Autodesk Inventor part; units mm, degrees
ref_plane "YZ Plane" through (0, 0, 0) normal (1, 0, 0) x (0, 1, 0)
ref_plane "XZ Plane" through (0, 0, 0) normal (0, 1, 0) x (-1, 0, 0)
ref_plane "XY Plane" through (0, 0, 0) normal (0, 0, 1) x (1, 0, 0)
sketch "Sketch1" plane through (0, 0, 0) normal (1, 0, 0) x (0, 1, 0)
  circle A0 centre (0, 0) radius 4.7625
  line L0 (0, 0) -> (-76.2, 0) construction
  circle A1 centre (0, 0) radius 19.05
  line L1 (-4.7625, 18.4451) -> (-76.2, 0)
  line L2 (-76.2, 0) -> (-76.2, -114.3)
  circle A2 centre (0, 0) radius 76.2 construction
  line L3 (-76.2, -114.3) -> (-41.275, -114.3)
  line L4 (-41.275, -114.3) -> (-41.275, -69.85)
  line L5 (-41.275, -69.85) -> (-76.2, -49.686)
  line L6 (-41.275, -69.85) -> (13.6667, -13.2712)
  line L7 (-52.6181, -63.301) -> (-7.9567, -17.3088)
  line L8 (-66.675, -9.525) -> (-66.675, -55.1853)
  line L9 (-46.0375, -78.0989) -> (-76.2, -60.6846)
  line L10 (-46.0375, -78.0989) -> (-46.0375, -106.3625)
  line L11 (-46.0375, -106.3625) -> (-69.85, -106.3625)
  line L12 (-69.85, -106.3625) -> (-69.85, -64.3507)
  line L13 (-66.675, -9.525) -> (-64.7847, -9.525)
  line L14 (-64.7847, -9.525) -> (-16.4978, -9.525)
  line L15 (-76.2, 0) -> (-41.275, 0)
  line L16 (-41.275, 0) -> (-41.275, 25.4) construction
  line L17 (-41.275, 25.4) -> (-76.2, 25.4) construction
  line L18 (-76.2, 25.4) -> (-76.2, 0)
  line L19 (-41.275, 0) -> (-76.2, 25.4)
  point P0 (-50.4255, 6.6549)
  dimension "d0" = 9.525
  dimension "d1" = 76.2
  dimension "d2" = 38.1
  dimension "d3" = 114.3
  dimension "d4" = 152.4
  dimension "d5" = 34.925
  dimension "d6" = 44.45
  dimension "d7" = 60
  dimension "d9" = 12.7
  dimension "d10" = 9.525
  dimension "d11" = 9.525
  dimension "d12" = 7.9375
  dimension "d13" = 6.35
  dimension "d14" = 4.7625
  dimension "d17" = 9.525
  dimension "d19" = 34.925
  dimension "d20" = 25.4
extrude "Extrusion1" add sketch "Sketch1" along normal blind 6.35 contours A1 | A1 L14 L13 L8 L5 L2 L15 L19 L1 | L6 L5 L7 A1 | L19 L15 L1 | L1 L18 L19 | L4 L3 L2 L5
fillet "Fillet1" radius 6.35 10 edges at (3.175, -7.9567, -17.3088) (3.175, -16.4978, -9.525) (3.175, -52.6181, -63.301) (3.175, -66.675, -9.525) (3.175, -66.675, -55.1853) (3.175, -69.85, -64.3507) (3.175, -46.0375, -78.0989) (3.175, -46.0375, -106.3625) (3.175, -69.85, -106.3625) (3.175, -41.275, -69.85)
fillet "Fillet2" radius 6.35 2 edges at (3.175, -76.2, 25.4) (3.175, -50.4255, 6.6549)
sketch "Sketch2" plane through (6.35, 0, 0) normal (1, 0, 0) x (0, 0, -1)
  circle A0 centre (0, 0) radius 4.7625
  circle A1 centre (0, 0) radius 11.1125
  dimension "d24" = 22.225
extrude "Extrusion2" cut sketch "Sketch2" against normal blind 1.5875 contours A0 | A1
equation "\"d9\" = d8"
properties part number "Upright" material "Aluminum 6061"
Work out the finished part from the listing and answer in its coordinate system (mm). A direction names the side the tool comes from. Round coordinates to 2 decimals unless told otherwise and drop trailing zeros. Order: outer loops, then holes, each group sorted by start corner. A loop starts at its lowest first (then second) coordinate and runs counter-clockwise, first axis right, second up. Notation, with made-up numbers: M 20,80 L 76,80 A25 cw 76,97 Z; hole C -27.5,-14.5 d9. An arc over 180 degrees is marked long. Put each result on its own line as item: value. Start each with the question number.
Q1. Section D-D, the plane z = 0 is taken. Write down the section's boundary in (x, y), and give its area (3 significant figures).
Q2. Straight lines are drawn through the part: L1, parallel to Z at x = 1.75, y = -64; L2, parallel to Y at x = 5.1, z = 0; L3, parallel to Z at x = 5.5, y = -57.5 (1 decimal). For each, find the intervals that lie inside material, in ascending order. Write a range as [from, to].
Q3. Section C-C, the plane x = 1 is taken. Give the number of separate pieces and of enclosed holes in the cut face, and give its area (3 significant figures).
Q4. Section B-B, the plane y = 0 is taken. Write down the section's boundary in (x, z).
Q5. Flat-ended cylindrical pins translate along their axes: pin 1 (3 mm diameter, centred on x = 5, y = -62, fed in from +Z); pin 2 (3 mm diameter, centred on x = 5.5, z = -97.5, fed in from +Y) (3 decimals); pin 3 (3 mm diameter, centred on x = 2, y = -57, fed in from +Z). Find the tip coordinate at first contact, or state that the pin passes through.
Q6. For a pull along Y with two mould halves and no side action, classify faces 1 (the cylindrical face through (3.219, -40.796, -70.007)), 2 (the flat face through (3.13, -31.41, -41.46)) as pulls with the +Y half, pulls with the -Y half, needs draft (parallel to the pull), parting line crosses it, or undercut.
Q7. A tool of negligible diameter and unlimited length cuts with its end or side. For faces 3 (the cylindrical face through (3.219, -52.911, -61.626)), 4 (the flat face through (3.131, -25.845, 13.002)), 5 (the flat face through (3, -41.275, -94)), from which of +Z, -Z, +X, -X, +Y, -Y can it reach the whole face along a straight path? Write none if from no direction.
Findings below:
1. outline: M 0,-76.2 L 6.35,-76.2 L 6.35,-11.11 L 4.76,-11.11 L 4.76,-4.76 L 0,-4.76 Z; M 0,4.76 L 4.76,4.76 L 4.76,11.11 L 6.35,11.11 L 6.35,19.05 L 0,19.05 Z
1. area: 524 mm^2
2. L1: z = [-114.3, -106.34], [-69.02, -56.7], [-10.7, 16.53]
2. L2: y = [-76.2, -11.11], [11.11, 19.05]
2. L3: z = [-114.3, -106.4], [-71.5, -60.5], [-9.5, 11.8]
3. separate pieces: 1
3. enclosed holes: 3
3. area: 4,790 mm^2
4. outline: M 0,-27.35 L 6.35,-27.35 L 6.35,-11.11 L 4.76,-11.11 L 4.76,-4.76 L 0,-4.76 Z; M 0,4.76 L 4.76,4.76 L 4.76,11.11 L 6.35,11.11 L 6.35,19.05 L 0,19.05 Z
5. pin 1: stops at z = 16.16
5. pin 2: stops at y = -41.275
5. pin 3: stops at z = 12.53
6. face 1: pulls with the +Y half
6. face 2: undercut
7. face 3: +X, -X
7. face 4: +Z, +X, -X
7. face 5: -Z, +X, -X, +Y
